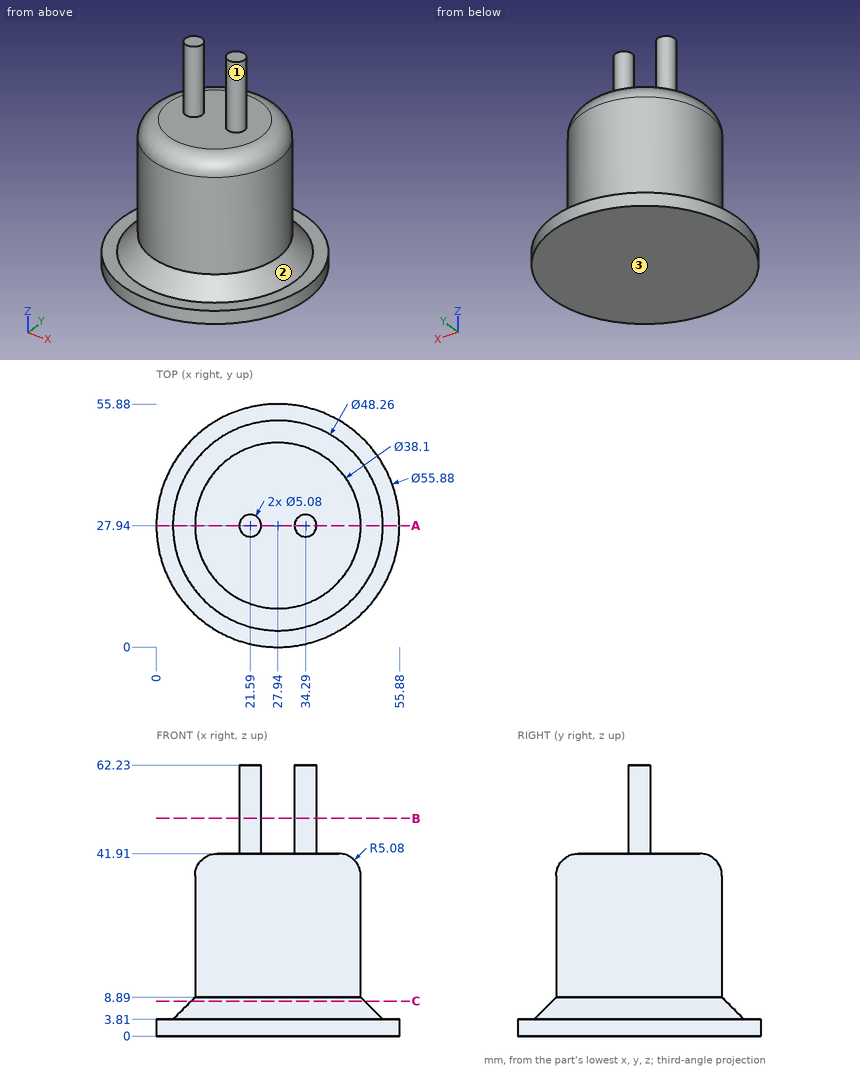
Study the drawing (mm; zero at the part's minimum x, y, z) and answer. Coordinates: 2 decimals unless noted, no trailing zeros. Write each loop counter-clockwise with the first axis right and the second up, starting at its lowest first coordinate (ties: lowest second). Pieces come first, ordered by that corner, then holes. Notation, with made-up numbers: M 49.25,-20 L 98.25,-20 A27 ccw 98.25,12 Z; hole C 7.25,46 d1. An arc over 180 degrees is marked long. Use one line per item in the form item = value.
Item 1: Given P1, Ø1, axis at x = 17.5, z = 18, coming from the +Y side; P2, Ø10, axis at x = 16, z = 28, coming from the +Y side; P3, Ø17, axis at x = 20, y = 14.5, coming from the +Z side, each flat-ended and moving along its own axis, determine where each tip first touches the part or whether it passes through.
Model answer:
P1 = 44.19
P2 = 45.68
P3 = 41.91
Item 2: Find the intervals of material crossed by probe 1 along Z at (x, y) = (24, 31); probe 2 along Y at (x, z) = (23.5, 47); probe 3 along X at (y, z) = (43.5, 19), in increasing order.
Model answer:
probe_1 = 0 to 41.91
probe_2 = 26.27 to 29.61
probe_3 = 16.95 to 38.93
Item 3: Find section B-B, the plane z = 50. Give the vertices of the cut face in (x, y), plus the area to 3 significant figures.
Model answer:
outline = C 21.59,27.94 d5.08; C 34.29,27.94 d5.08
area = 40.5 mm2
Item 4: The mould has two halves that part along X. Classify the marked faces 1, 2 and 3: released by +X, released by -X, zero draft, split by the parting line, or undercut.
Model answer:
face_1 = undercut
face_2 = split by the parting line
face_3 = zero draft
Item 5: Find section C-C, the plane z = 8. Give the vertices of the cut face in (x, y).
Model answer:
outline = C 27.94,27.94 d39.88
Item 6: Find section A-A, the plane y = 27.94. Give the vertices of the cut face in (x, z), plus the area to 3 significant figures.
Model answer:
outline = M 0,0 L 55.88,0 L 55.88,3.81 L 52.07,3.81 L 46.99,8.89 L 46.99,36.83 A5.08 ccw 41.91,41.91 L 36.83,41.91 L 36.83,62.23 L 31.75,62.23 L 31.75,41.91 L 24.13,41.91 L 24.13,62.23 L 19.05,62.23 L 19.05,41.91 L 13.97,41.91 A5.08 ccw 8.89,36.83 L 8.89,8.89 L 3.81,3.81 L 0,3.81 Z
area = 1,890 mm2
